Geometry: see drawing. Coordinates: mm, zero at the bounding-box minimum. A direction names the side the tool comes from. Give positions to 0.01 mm unless a question says otherwise; leave off trailing zeros. Loops run counter-clockwise (first coordinate to the right, second up) from the corner with the lowest first, then second, coordinate; pieces in that order, holes last. Notation, with made-up numbers: (49.5, -18.75) -> (103.5, -18.75) arc R4 cw to (103.5, -11.75) -> close; hole circle Ø9 at (-16.5, 77). An arc over 180 degrees is marked (long way). Return JSON: item names as keys, results as strings. Group by question number.
(1) Pin query (flat end, axial travel): pin 1 (16.5 mm diameter, centred on x = 111, y = 43, fed in from +Z); pin 2 (12.5 mm diameter, centred on y = 35.5, z = 42.5, fed in from +X). Return the tip coordinate at first contact, or that it passes through.
(2) Cut plane D-D on y = 4. Return loops of the section in (x, z).
(3) Cut plane A-A on x = 48.5. Return loops of the section in (y, z), then the cut area to 3 significant figures.
(4) Ray query, line 1 (X direction, y = 22, z = 11.5); line 2 (Y direction, x = 37, z = 22.5); line 3 (X direction, y = 50.5, z = 38). Return the intervals inside material, ascending. Write a range as from..to.
(5) Cut plane B-B on y = 26. Return loops of the section in (x, z), then the cut area to 3 significant figures.
(6) Cut plane C-C on z = 11.5. Return loops of the section in (x, y).
(7) Draft query along Y for the marked faces 1, 2 and 3. Return one class per face: released by +Y, released by -Y, zero draft, split by the parting line, or undercut.
(8) Access query for the marked faces 4, 5 and 6. Directions: +Z, -Z, +X, -X, +Y, -Y. A direction counts if a zero-diameter tool reaches every point of the face in a straight line with its end or side. Return the directions, or none.
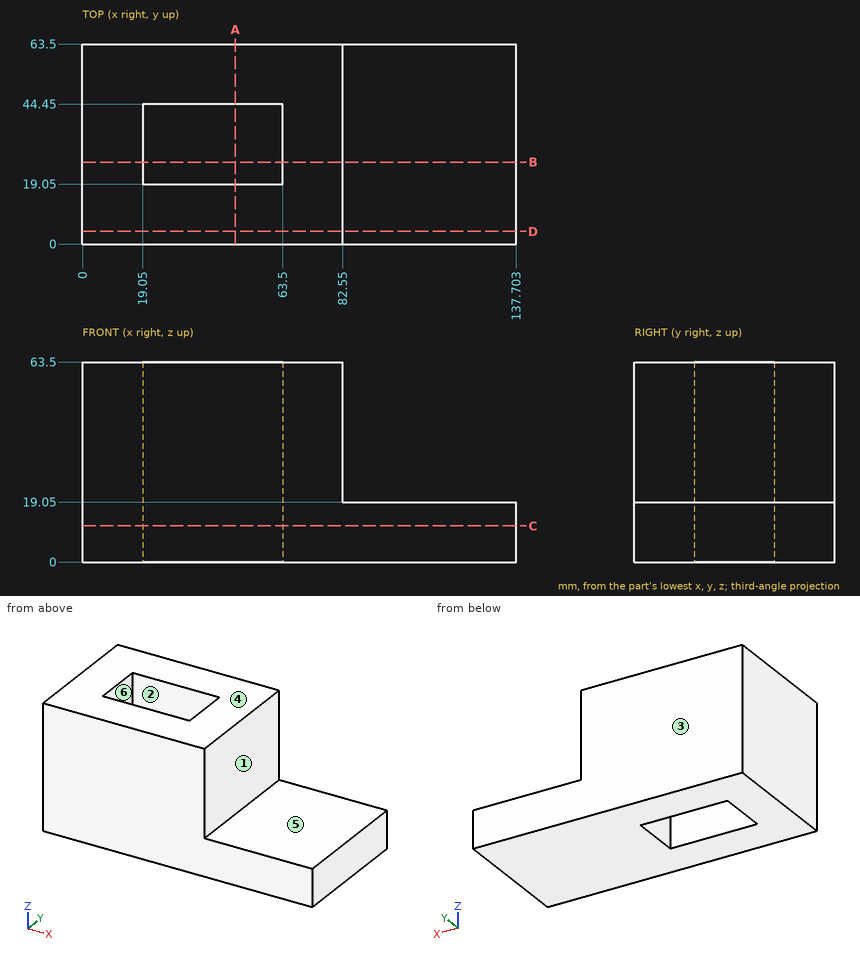
Answers:
{
 "1": {"pin 1": "z = 19.05", "pin 2": "x = 82.55"},
 "2": {"outline": "(0, 0) -> (137.7, 0) -> (137.7, 19.05) -> (82.55, 19.05) -> (82.55, 63.5) -> (0, 63.5) -> close"},
 "3": {"outline": "(0, 0) -> (19.05, 0) -> (19.05, 63.5) -> (0, 63.5) -> close; (44.45, 0) -> (63.5, 0) -> (63.5, 63.5) -> (44.45, 63.5) -> close", "area": "2,420 mm²"},
 "4": {"line 1": "0..19.05, 63.5..137.7", "line 2": "0..19.05, 44.45..63.5", "line 3": "0..82.55"},
 "5": {"outline": "(0, 0) -> (19.05, 0) -> (19.05, 63.5) -> (0, 63.5) -> close; (63.5, 0) -> (137.7, 0) -> (137.7, 19.05) -> (82.55, 19.05) -> (82.55, 63.5) -> (63.5, 63.5) -> close", "area": "3,470 mm²"},
 "6": {"outline": "(0, 0) -> (137.7, 0) -> (137.7, 63.5) -> (0, 63.5) -> close; hole (19.05, 19.05) -> (63.5, 19.05) -> (63.5, 44.45) -> (19.05, 44.45) -> close"},
 "7": {"face 1": "zero draft", "face 2": "undercut", "face 3": "released by +Y"},
 "8": {"face 4": "+Z, +X, -X, +Y, -Y", "face 5": "+Z, +X, +Y, -Y", "face 6": "+Z, -Z"}
}
